Geometry check sheet. Reference: the model listing, model coordinates, mm. A direction names the side the tool comes from. Coordinates: 2 decimals unless noted, no trailing zeros. Order: outer loops, then holes, each group sorted by start corner. A loop starts at its lowest first (then second) coordinate and runs counter-clockwise, first axis right, second up. Notation, with made-up numbers: M 33.25,16 L 41.25,16 A22 ccw 41.25,27 Z; hole C 25.5,89.25 d2. An arc over 180 degrees is marked long. Use CSV: the item, a comma, the result in double quotes. Start each with the question number.
```python
from build123d import *

# Parameters (mm, degrees)
SKETCH1_W                = 30
SKETCH1_H                = 45
SKETCH1_R                = 1.6
BOSS_EXTRUDE3_DEPTH      = 5
SKETCH2_W                = 64
SKETCH2_H                = 27.1
SKETCH2_W_2              = 30
BOSS_EXTRUDE4_DEPTH      = 35
BOSS_EXTRUDE4_DEPTH_BACK = 1.7
SKETCH3_W                = 4
SKETCH3_H                = 24.6
SKETCH3_W_2              = 5
SKETCH3_H_2              = 27.1
SKETCH3_W_3              = 2
BOSS_EXTRUDE5_DEPTH      = 3.3
CUT_EXTRUDE2_DEPTH       = 60
SKETCH6_R                = 1.4
CUT_EXTRUDE3_DEPTH       = 39
SKETCH7_W                = 27.1
SKETCH7_H                = 36.7
CUT_EXTRUDE4_DEPTH       = 2.6
CUT_EXTRUDE5_DEPTH       = 15
CUT_EXTRUDE5_DEPTH_BACK  = 15
CUT_EXTRUDE6_DEPTH       = 9.4
CUT_EXTRUDE7_DEPTH       = 37.05
FILLET1_R                = 2


with BuildPart() as part:
    # Sketch1 → Boss-Extrude3 (new body)
    with BuildSketch(Plane(origin=(0, 0, 0), x_dir=(1, 0, 0), z_dir=(0, 1, 0))):
        Rectangle(SKETCH1_W, SKETCH1_H)
        with Locations((-10, 17.5)):
            Circle(SKETCH1_R, mode=Mode.SUBTRACT)
        with Locations((10, 17.5)):
            Circle(SKETCH1_R, mode=Mode.SUBTRACT)
        with Locations((10, -17.5)):
            Circle(SKETCH1_R, mode=Mode.SUBTRACT)
        with Locations((-10, -17.5)):
            Circle(SKETCH1_R, mode=Mode.SUBTRACT)
    extrude(amount=BOSS_EXTRUDE3_DEPTH)

    # Sketch2 → Boss-Extrude4 (add, two sides)
    with BuildSketch(Plane(origin=(0, 5, 0), x_dir=(1, 0, 0), z_dir=(0, 1, 0))) as boss_extrude4_sk:
        with Locations((-47, 0)):
            Rectangle(SKETCH2_W, SKETCH2_H)
        Rectangle(SKETCH2_W_2, SKETCH2_H)
    extrude(amount=BOSS_EXTRUDE4_DEPTH)
    extrude(boss_extrude4_sk.sketch, amount=-BOSS_EXTRUDE4_DEPTH_BACK)

    # Sketch3 → Boss-Extrude5 (add)
    with BuildSketch(Plane.XZ.offset(-3.3)):
        with Locations((-38, -1.25)):
            Rectangle(SKETCH3_W, SKETCH3_H)
        with Locations((-17.5, 0)):
            Rectangle(SKETCH3_W_2, SKETCH3_H_2)
        with Locations((-24, 0)):
            Rectangle(SKETCH3_W_3, SKETCH3_H_2)
    extrude(amount=BOSS_EXTRUDE5_DEPTH)

    # Sketch5 → Cut-Extrude2 (cut)
    with BuildSketch(Plane.ZY.offset(79)):
        Polygon((-8.55, 40), (13.55, 8.3), (13.55, 40), align=None)
    extrude(amount=-CUT_EXTRUDE2_DEPTH, mode=Mode.SUBTRACT)

    # Sketch6 → Cut-Extrude3 (cut)
    with BuildSketch(Plane(origin=(0, 9.071537199, 13.012114445), x_dir=(1, 0, 0), z_dir=(0, 0.571898215, 0.820324589))):
        with Locations((-62, 26.38109329)):
            Circle(SKETCH6_R)
        with Locations((-42, 26.38109329)):
            Circle(SKETCH6_R)
        with Locations((-41.999995471, 10.38109329)):
            Circle(SKETCH6_R)
        with Locations((-61.999995471, 10.38109329)):
            Circle(SKETCH6_R)
    extrude(amount=-CUT_EXTRUDE3_DEPTH, mode=Mode.SUBTRACT)

    # Sketch7 → Cut-Extrude4 (cut)
    with BuildSketch(Plane.ZY.offset(79)):
        with Locations((0, 21.65)):
            Rectangle(SKETCH7_W, SKETCH7_H)
    extrude(amount=-CUT_EXTRUDE4_DEPTH, mode=Mode.SUBTRACT)

    # Sketch10 → Cut-Extrude5 (cut, two sides)
    with BuildSketch(Plane.ZY.offset(52)) as cut_extrude5_sk:
        Polygon((-13.55, 35), (-13.55, 3.3), (8.55, 3.3), (8.55, 6.729131215), (-11.159343853, 35), align=None)
    extrude(amount=CUT_EXTRUDE5_DEPTH, mode=Mode.SUBTRACT)
    extrude(cut_extrude5_sk.sketch, amount=-CUT_EXTRUDE5_DEPTH_BACK, mode=Mode.SUBTRACT)

    # Sketch11 → Cut-Extrude6 (cut)
    with BuildSketch(Plane.ZY.offset(76.4)):
        Polygon((-13.55, 35), (-13.55, 3.3), (8.55, 3.3), (8.55, 6.729131215), (-11.159343853, 35), align=None)
    extrude(amount=-CUT_EXTRUDE6_DEPTH, mode=Mode.SUBTRACT)

    # Sketch12 → Cut-Extrude7 (cut, through all)
    with BuildSketch(Plane.XY.offset(13.55)):
        Polygon((-19, 40), (15, 5), (15, 40), align=None)
    extrude(amount=-CUT_EXTRUDE7_DEPTH, mode=Mode.SUBTRACT)

    # Fillet1
    fillet1_edges = [part.edges().sort_by_distance(p)[0] for p in [
        (-37, 20.864565607, -1.304671927),
    ]]
    fillet(fillet1_edges, radius=FILLET1_R)


solid = part.part
```
1) Material ranges on line 1 along Z through (x, y) = (10, 1.65); line 2 along X through (y, z) = (1.7, -17.5); line 3 along X through (y, z) = (2, -17), recorded low to high.
2) Section check D-D on z = 6. State how many separate pieces and enclosed holes the cut face has, then the cut area to 3 significant figures.
3) Section check A-A on z = -17.5. Record the boundary of the cut face in (x, y).
4) Gauge pin test, flat ends, axial feed: P1, Ø2.5, axis at y = 1, z = 1, coming from the -X side; P2, Ø1.5, axis at x = -36, y = 19.5, coming from the -Z side; P3, Ø3, axis at y = 32.5, z = 12, coming from the -X side. Record the tip position at first contact, or that the pin passes through.
5) Set-up check for faces 1 (the face through (-37.57, 20.15, -1.54)), 2 (the face through (-40, 2, -1)), 3 (the face through (-15, 2, -18)), 4 (the face through (-40.665, 29.648, -4.338)): record each of +Z, -Z, +X, -X, +Y, -Y from which the full face is reachable in a straight line by a thin tool's end or side.
6) Draft check along X on faces 5 (the face through (-15, 2, 18)), 6 (the face through (-56, 5, 8.55)), 7 (the face through (-23, 2, 0)). Enter one of: +X half, -X half, draft (parallel to the pull), parting line (faces both ways), or undercut.
7) Section check B-B on x = -56.5. Record the boundary of the cut face in (y, z).
8) Section check C-C on x = 10. Record the boundary of the cut face in (y, z), then the cut area to 3 significant figures.
Results are:
1,line 1,"z = -22.5 to -19.1, -15.9 to 15.9, 19.1 to 22.5"
1,line 2,"x = -15 to -11.6, -8.4 to 8.4, 11.6 to 15"
1,line 3,"x = -15 to -11.52, -8.48 to 8.48, 11.52 to 15"
2,separate pieces,"1"
2,enclosed holes,"2"
2,area,"1,400 mm²"
3,outline,"M -15,0 L -11.6,0 L -11.6,5 L -15,5 Z; M -8.4,0 L 8.4,0 L 8.4,5 L -8.4,5 Z; M 11.6,0 L 15,0 L 15,5 L 11.6,5 Z"
4,P1,"stops at x = -40"
4,P2,"stops at z = -13.55"
4,P3,"stops at x = -19"
5,face 1,"-Z, -X"
5,face 2,"+Z, -Z, -X, -Y"
5,face 3,"-Z, -X, +Y, -Y"
5,face 4,"none"
6,face 5,"-X half"
6,face 6,"draft"
6,face 7,"undercut"
7,outline,"M 3.3,8.55 L 6.73,8.55 L 35,-11.16 L 35,-13.55 L 40,-13.55 L 40,-8.55 L 8.3,13.55 L 3.3,13.55 Z"
8,outline,"M 0,-22.5 L 5,-22.5 L 5,-19.1 L 0,-19.1 Z; M 0,-15.9 L 5,-15.9 L 5,-13.55 L 10.15,-13.55 L 10.15,13.55 L 5,13.55 L 5,15.9 L 0,15.9 Z; M 0,19.1 L 5,19.1 L 5,22.5 L 0,22.5 Z"
8,area,"332 mm²"
